CAD build for the part. Positions are in the model's coordinates, mm. Round coordinates to 2 decimals unless told otherwise and drop trailing zeros. Write each loop counter-clockwise with the first axis right and the second up, starting at its lowest first coordinate (ties: lowest second). Pieces come first, ordered by that corner, then holes. Notation, with made-up numbers: (59, 51) - (109, 51) arc R23 cw to (109, 79) - close; hole circle Ø10 at (-14, 28). An arc over 180 degrees is marked (long way). Put each result on its own line as item: value. Start each with the question number.
Item 1: Cut at A-A (x = 28). Give the cut face in (y, z), and give its area (3 significant figures).
Item 2: Cut at B-B (z = -151). Give the cut face in (x, y), and give its area (3 significant figures).
Item 3: Drill centre lines: line 1 (X direction, y = -7.75, z = -182); line 2 (X direction, y = -15.75, z = -130); line 3 (Z direction, x = -198, y = -5.5). Where is each one in solid material? Low to high. Write a range as from..to.
Item 4: Cut at C-C (y = -12). Count the separate pieces of the cut face and the enclosed holes in it, and give its area (3 significant figures).
```python
from build123d import *

# Parameters (mm, degrees)
F0_W     = 500
F0_H     = 450
F0_R     = 2.75
F0_W_2   = 45
F0_H_2   = 142.5
F0_W_3   = 142.5
F0_H_3   = 45
F1_DEPTH = 20


with BuildPart() as f1:
    # F0 (on Front) → F1 (new body)
    with BuildSketch(Plane.XZ):
        with Locations((-30, 0)):
            Rectangle(F0_W, F0_H)
        with Locations((-230, -182)):
            Circle(F0_R, mode=Mode.SUBTRACT)
        with Locations((-198, -182)):
            Circle(F0_R, mode=Mode.SUBTRACT)
        with Locations((90, -182)):
            Circle(F0_R, mode=Mode.SUBTRACT)
        with Locations((122, -182)):
            Circle(F0_R, mode=Mode.SUBTRACT)
        with Locations((-230, 204)):
            Circle(F0_R, mode=Mode.SUBTRACT)
        with Locations((-198, 204)):
            Circle(F0_R, mode=Mode.SUBTRACT)
        Polygon((-165, 22.5), (-165, 165), (-22.5, 165), (22.5, 165), (165, 165), (165, 22.5), (165, -22.5), (165, -165), (22.5, -165), (-22.5, -165), (-165, -165), (-165, -22.5), align=None, mode=Mode.SUBTRACT)
        with Locations((90, 204)):
            Circle(F0_R, mode=Mode.SUBTRACT)
        with Locations((122, 204)):
            Circle(F0_R, mode=Mode.SUBTRACT)
        with Locations((0, 93.75)):
            Rectangle(F0_W_2, F0_H_2)
        with Locations((-93.75, 0)):
            Rectangle(F0_W_3, F0_H_3)
        with Locations((0, -93.75)):
            Rectangle(F0_W_2, F0_H_2)
        with Locations((93.75, 0)):
            Rectangle(F0_W_3, F0_H_3)
        Rectangle(F0_W_2, F0_H_3)
    extrude(amount=F1_DEPTH)


solid = f1.part
```
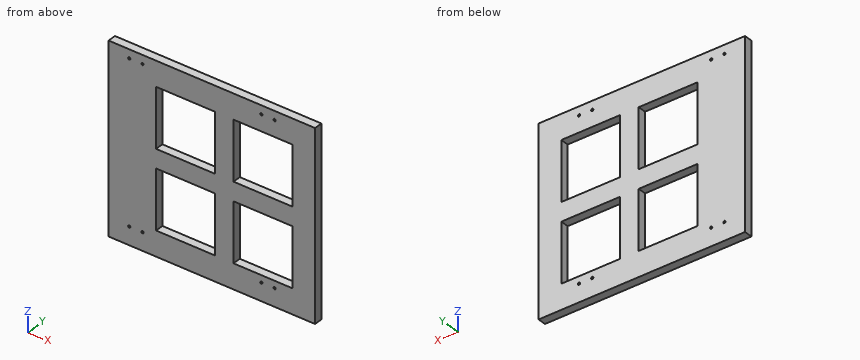
Output values:
1. outline: (-20, -225) - (0, -225) - (0, -165) - (-20, -165) - close; (-20, -22.5) - (0, -22.5) - (0, 22.5) - (-20, 22.5) - close; (-20, 165) - (0, 165) - (0, 225) - (-20, 225) - close
1. area: 3,300 mm2
2. outline: (-280, -20) - (-165, -20) - (-165, 0) - (-280, 0) - close; (-22.5, -20) - (22.5, -20) - (22.5, 0) - (-22.5, 0) - close; (165, -20) - (220, -20) - (220, 0) - (165, 0) - close
2. area: 4,300 mm2
3. line 1: -280..-232.75, -227.25..-200.75, -195.25..87.25, 92.75..119.25, 124.75..220
3. line 2: -280..-165, -22.5..22.5, 165..220
3. line 3: -225..-184.75, -179.25..201.25, 206.75..225
4. separate pieces: 1
4. enclosed holes: 12
4. area: 144,000 mm2
